Model file for the job. Use its own axes, mm. A direction names the side the tool comes from. Give positions to 0.01 mm unless a question says otherwise; leave off trailing zeros. Order: outer loops, then holes, each group sorted by start corner. A loop starts at its lowest first (then second) coordinate and runs counter-clockwise, first axis right, second up. Notation, with made-up numbers: (-4, 12.5) -> (1, 12.5) arc R13 cw to (1, 36.5) -> close; hole circle Ø11 at (1.25, 89). An arc over 180 degrees is marked (long way). Answer in a Markdown table with one row per item. Add a question column.
from build123d import *

# Parameters (mm, degrees)
SKETCH_2_W      = 30
SKETCH_2_H      = 30
SKETCH_2_R      = 1.45
EXTRUDE_1_DEPTH = 1.5
FILLET_1_R      = 2.4


with BuildPart() as part:
    # Эскиз1 → Повернуть1 (revolve)
    with BuildSketch(Plane.XY):
        Polygon((0, 0), (0, 15), (71, 15), (71, 11), (72.5, 11), (72.5, 4.511822107), (74, 4.511822107), (74, 2), (80, 2), (84.5, 2), (84.5, 0), align=None)
    revolve(axis=Axis((0, 0, 0), (1, 0, 0)))

    # Эскиз2 → Бобышка-Вытянуть1 (add)
    with BuildSketch(Plane(origin=(71, 0, 0), x_dir=(0, 0, -1), z_dir=(1, 0, 0))):
        Rectangle(SKETCH_2_W, SKETCH_2_H)
        with Locations((-12.6, 12.6)):
            Circle(SKETCH_2_R, mode=Mode.SUBTRACT)
        with Locations((12.6, 12.6)):
            Circle(SKETCH_2_R, mode=Mode.SUBTRACT)
        with Locations((12.6, -12.6)):
            Circle(SKETCH_2_R, mode=Mode.SUBTRACT)
        with Locations((-12.6, -12.6)):
            Circle(SKETCH_2_R, mode=Mode.SUBTRACT)
    extrude(amount=-EXTRUDE_1_DEPTH)

    # Скругление1
    fillet_1_edges = [part.edges().sort_by_distance(p)[0] for p in [
        (70.25, -15, -15),
        (70.25, -15, 15),
        (70.25, 15, 15),
        (70.25, 15, -15),
    ]]
    fillet(fillet_1_edges, radius=FILLET_1_R)


solid = part.part
Item 1: Which spindle directions (+Z, -Z, +X, -X, +Y, -Y) get a long thin tool onto all of the face, cutting with end or side? Do faces 1 (the flat face through (69.5, 11, -11)), 2 (the flat face through (71, 10, 7)), 3 (the cylindrical face through (35.236, -14.985, 0.66)). Say none if no direction does.
Item 2: Saw through at A-A on x = 78.5. List the corners of the cut face in (y, z), plus the area to 3 significant figures.
Item 3: Saw through at C-C on y = 8.5. List the corners of the cut face in (x, z).
Item 4: Two-plate mould, pull along Y, no slides. Class faces 4 (the cylindrical face through (70.26, 13.58, 13.67)), 5 (the flat face through (70, 15, 0)), 6 (the flat face through (84.5, 0, 0)): pulls with the +Y half, pulls with the -Y half, needs draft (parallel to the pull), parting line crosses it, or undercut.
Item 5: Wall check: line 1 (Y direction, x = 69.9, z = -12.6); line 2 (Y direction, x = 70, z = 12). Give the ranges that are in metal, low to high.
Item 6: Saw through at B-B on z = 5.5. List the corners of the cut face in (x, y), plus the area to 3 significant figures.
Item 7: Saw through at D-D on x = 63. List the corners of the cut face in (y, z), plus the area to 3 significant figures.
Item 8: Pin check, flat tips, straight feed: pin 1 Ø16.5 at (y, z) = (10, 10.5) entering from -X; pin 2 Ø3 at (x, y) = (24.5, -3) entering from -Z; pin 3 Ø12 at (x, z) = (9, 10.5) entering from -Y; pin 4 Ø1.5 at (x, y) = (49, -4.5) entering from -Z. Stop position of each tip, or through.
Evaluation:
| question | item | result |
|---|---|---|
| 1 | face 1 | -Z, -X, +Y |
| 1 | face 2 | +X |
| 1 | face 3 | -X |
| 2 | outline | circle Ø4 at (0, 0) |
| 2 | area | 12.6 mm2 |
| 3 | outline | (0, -12.36) -> (69.5, -12.36) -> (69.5, -15) -> (71, -15) -> (71, -6.98) -> (72.5, -6.98) -> (72.5, 6.98) -> (71, 6.98) -> (71, 15) -> (69.5, 15) -> (69.5, 12.36) -> (0, 12.36) -> close |
| 4 | face 4 | undercut |
| 4 | face 5 | pulls with the +Y half |
| 4 | face 6 | needs draft |
| 5 | line 1 | y = -15 to -14.05, -11.15 to 11.15, 14.05 to 15 |
| 5 | line 2 | y = -15 to -13.92, -11.28 to 11.28, 13.92 to 15 |
| 6 | outline | (0, -13.96) -> (69.5, -13.96) -> (69.5, -15) -> (71, -15) -> (71, -9.53) -> (72.5, -9.53) -> (72.5, 9.53) -> (71, 9.53) -> (71, 15) -> (69.5, 15) -> (69.5, 13.96) -> (0, 13.96) -> close |
| 6 | area | 2,010 mm2 |
| 7 | outline | circle Ø30 at (0, 0) |
| 7 | area | 707 mm2 |
| 8 | pin 1 | stops at x = 0 |
| 8 | pin 2 | stops at z = -14.92 |
| 8 | pin 3 | stops at y = -14.31 |
| 8 | pin 4 | stops at z = -14.52 |
